from build123d import *

# Parameters (mm, degrees)
SM_BASE_FLANGE_1_DEPTH     = 500
CHAMFER_2_SIZE             = 1
CUT_EXTRUDE_1_DEPTH        = 1012.596757607
PATTERN_CIRCULAR_1_COUNT   = 4
PATTERN_CIRCULAR_1_ANGLE   = 90
F_1_THE_OTHER_WAY_COUNT    = 4
F_1_THE_OTHER_WAY_ANGLE    = 90
CHAMFER_1_SIZE             = 3
HOLE_WIZARD_M61_AT_2_COUNT = 2
HOLE_WIZARD_M61_AT_2_PITCH = 150
HOLE_WIZARD_M61_AT_3_COUNT = 2
HOLE_WIZARD_M61_AT_3_PITCH = 300
HOLE_WIZARD_M61_AT_4_COUNT = 2
HOLE_WIZARD_M61_AT_4_PITCH = 450
HOLE_WIZARD_M61_AT_5_COUNT = 2
HOLE_WIZARD_M61_AT_5_PITCH = 600
HOLE_WIZARD_M61_AT_6_COUNT = 2
HOLE_WIZARD_M61_AT_6_PITCH = 750
HOLE_WIZARD_M61_AT_7_COUNT = 2
HOLE_WIZARD_M61_AT_7_PITCH = 900


# Sheet-metal steps are written as plain solids
with BuildPart() as part:
    # Sketch 2 → Базовая кромка1 (new, symmetric)
    with BuildSketch(Plane.XY):
        with BuildLine():
            Line((100, 95), (100, 0))
            ThreePointArc((100, 0), (0, -100), (-100, 0))
            Line((-100, 0), (-100, 95))
            Line((-100, 95), (-108, 95))
            Line((-108, 95), (-108, 0))
            ThreePointArc((-108, 0), (0, -108), (108, 0))
            Line((108, 0), (108, 95))
            Line((108, 95), (100, 95))
        make_face()
    extrude(amount=SM_BASE_FLANGE_1_DEPTH, both=True)

    # Фаска2
    chamfer_2_edges = [part.edges().sort_by_distance(p)[0] for p in [
        (100, 47.5, 500),
        (0, -100, 500),
        (-100, 47.5, 500),
        (0, -100, -500),
        (100, 47.5, -500),
        (-100, 47.5, -500),
    ]]
    chamfer(chamfer_2_edges, length=CHAMFER_2_SIZE)

    # Эскиз7 → Вырез-Вытянуть1 (cut, symmetric)
    with BuildSketch(Plane.XY.offset(500)):
        Polygon((0, 0), (-4, -102.92230079), (4, -102.92230079), align=None)
    cut_extrude_1 = extrude(amount=CUT_EXTRUDE_1_DEPTH, both=True, mode=Mode.SUBTRACT)

    # Круговой массив1: Вырез-Вытянуть1 ×4 about axis
    pattern_circular_1_axis = Axis((0, 0, 0), (0, 0, -1))
    for i in range(1, PATTERN_CIRCULAR_1_COUNT):
        add(cut_extrude_1.rotate(pattern_circular_1_axis, i * PATTERN_CIRCULAR_1_ANGLE / (PATTERN_CIRCULAR_1_COUNT - 1)), mode=Mode.SUBTRACT)

    # 1 the other way: Вырез-Вытянуть1 ×4 about axis
    f_1_the_other_way_axis = Axis((0, 0, 0), (0, 0, 1))
    for i in range(1, F_1_THE_OTHER_WAY_COUNT):
        add(cut_extrude_1.rotate(f_1_the_other_way_axis, i * F_1_THE_OTHER_WAY_ANGLE / (F_1_THE_OTHER_WAY_COUNT - 1)), mode=Mode.SUBTRACT)

    # Фаска1
    chamfer_1_edges = [part.edges().sort_by_distance(p)[0] for p in [
        (100, 95, 0),
        (-100, 95, 0),
    ]]
    chamfer(chamfer_1_edges, length=CHAMFER_1_SIZE)

    # Эскиз9 → Зенковка для винта с полупотайной головкой M61 (revolve, cut)
    with BuildSketch(Plane(origin=(-100, 75, 450), x_dir=(0, 0, -1), z_dir=(0, 1, 0))):
        Polygon((0, 0), (0, 18.982840043), (3.3, 17), (3.3, 3), (6.3, 0), align=None)
    hole_wizard_m61 = revolve(axis=Axis((-93.65, 75, 450), (-1, 0, 0)), mode=Mode.SUBTRACT)

    # Зенковка для винта с полупотайной головкой M61 at 2: Зенковка для винта с полупотайной головкой M61 ×2
    with Locations(*[(0, 0, -i * HOLE_WIZARD_M61_AT_2_PITCH) for i in range(1, HOLE_WIZARD_M61_AT_2_COUNT)]):
        add(hole_wizard_m61, mode=Mode.SUBTRACT)

    # Зенковка для винта с полупотайной головкой M61 at 3: Зенковка для винта с полупотайной головкой M61 ×2
    with Locations(*[(0, 0, -i * HOLE_WIZARD_M61_AT_3_PITCH) for i in range(1, HOLE_WIZARD_M61_AT_3_COUNT)]):
        add(hole_wizard_m61, mode=Mode.SUBTRACT)

    # Зенковка для винта с полупотайной головкой M61 at 4: Зенковка для винта с полупотайной головкой M61 ×2
    with Locations(*[(0, 0, -i * HOLE_WIZARD_M61_AT_4_PITCH) for i in range(1, HOLE_WIZARD_M61_AT_4_COUNT)]):
        add(hole_wizard_m61, mode=Mode.SUBTRACT)

    # Зенковка для винта с полупотайной головкой M61 at 5: Зенковка для винта с полупотайной головкой M61 ×2
    with Locations(*[(0, 0, -i * HOLE_WIZARD_M61_AT_5_PITCH) for i in range(1, HOLE_WIZARD_M61_AT_5_COUNT)]):
        add(hole_wizard_m61, mode=Mode.SUBTRACT)

    # Зенковка для винта с полупотайной головкой M61 at 6: Зенковка для винта с полупотайной головкой M61 ×2
    with Locations(*[(0, 0, -i * HOLE_WIZARD_M61_AT_6_PITCH) for i in range(1, HOLE_WIZARD_M61_AT_6_COUNT)]):
        add(hole_wizard_m61, mode=Mode.SUBTRACT)

    # Зенковка для винта с полупотайной головкой M61 at 7: Зенковка для винта с полупотайной головкой M61 ×2
    with Locations(*[(0, 0, -i * HOLE_WIZARD_M61_AT_7_PITCH) for i in range(1, HOLE_WIZARD_M61_AT_7_COUNT)]):
        add(hole_wizard_m61, mode=Mode.SUBTRACT)

    # Зеркальное отражение1: Зенковка для винта с полупотайной головкой M61 across plane
    add(hole_wizard_m61.mirror(Plane(origin=(0, 0, 0), x_dir=(0, 0, 1), z_dir=(1, 0, 0))), mode=Mode.SUBTRACT)

    # Зеркальное отражение1 copy 1 sketch → Зеркальное отражение1 copy 1 (revolve, cut)
    with BuildSketch(Plane(origin=(100, 75, 300), x_dir=(0, 0, -1), z_dir=(0, 1, 0))):
        Polygon((0, 0), (0, -18.982840043), (3.3, -17), (3.3, -3), (6.3, 0), align=None)
    revolve(axis=Axis((93.65, 75, 300), (-1, 0, 0)), mode=Mode.SUBTRACT)

    # Зеркальное отражение1 copy 2 sketch → Зеркальное отражение1 copy 2 (revolve, cut)
    with BuildSketch(Plane(origin=(100, 75, 150), x_dir=(0, 0, -1), z_dir=(0, 1, 0))):
        Polygon((0, 0), (0, -18.982840043), (3.3, -17), (3.3, -3), (6.3, 0), align=None)
    revolve(axis=Axis((93.65, 75, 150), (-1, 0, 0)), mode=Mode.SUBTRACT)

    # Зеркальное отражение1 copy 3 sketch → Зеркальное отражение1 copy 3 (revolve, cut)
    with BuildSketch(Plane(origin=(100, 75, 0), x_dir=(0, 0, -1), z_dir=(0, 1, 0))):
        Polygon((0, 0), (0, -18.982840043), (3.3, -17), (3.3, -3), (6.3, 0), align=None)
    revolve(axis=Axis((93.65, 75, 0), (-1, 0, 0)), mode=Mode.SUBTRACT)

    # Зеркальное отражение1 copy 4 sketch → Зеркальное отражение1 copy 4 (revolve, cut)
    with BuildSketch(Plane(origin=(100, 75, -150), x_dir=(0, 0, -1), z_dir=(0, 1, 0))):
        Polygon((0, 0), (0, -18.982840043), (3.3, -17), (3.3, -3), (6.3, 0), align=None)
    revolve(axis=Axis((93.65, 75, -150), (-1, 0, 0)), mode=Mode.SUBTRACT)

    # Зеркальное отражение1 copy 5 sketch → Зеркальное отражение1 copy 5 (revolve, cut)
    with BuildSketch(Plane(origin=(100, 75, -300), x_dir=(0, 0, -1), z_dir=(0, 1, 0))):
        Polygon((0, 0), (0, -18.982840043), (3.3, -17), (3.3, -3), (6.3, 0), align=None)
    revolve(axis=Axis((93.65, 75, -300), (-1, 0, 0)), mode=Mode.SUBTRACT)

    # Зеркальное отражение1 copy 6 sketch → Зеркальное отражение1 copy 6 (revolve, cut)
    with BuildSketch(Plane(origin=(100, 75, -450), x_dir=(0, 0, -1), z_dir=(0, 1, 0))):
        Polygon((0, 0), (0, -18.982840043), (3.3, -17), (3.3, -3), (6.3, 0), align=None)
    revolve(axis=Axis((93.65, 75, -450), (-1, 0, 0)), mode=Mode.SUBTRACT)


solid = part.part
The listing builds one solid part. Answer for the finished solid, in the listing's coordinates (mm). A direction names the side the tool comes from. Round coordinates to 2 decimals unless told otherwise and drop trailing zeros. Order: outer loops, then holes, each group sorted by start corner. A loop starts at its lowest first (then second) coordinate and runs counter-clockwise, first axis right, second up. Notation, with made-up numbers: (-23.5, 49.5) - (19.5, 49.5) arc R25 ccw to (19.5, 73.5) - close; hole circle Ø6 at (28, -19.5). An arc over 180 degrees is marked (long way). Write item = value, one per line. Start each with the question number.
1) Straight lines are drawn through the part: L1, parallel to X at y = 85.5, z = 85.5; L2, parallel to Y at x = -3.5, z = -127.5; L3, parallel to X at y = -88, z = -88.5. For each, find the intervals that lie inside material, in ascending order.
2) For faces 5 (the flat face through (31.5, -96.2, 500)), 6 (the conical face through (71.1, -70.6, 499.2)), 7 (the conical face through (71.1, -70.6, -499.2)), 8 (the flat face through (-100, 47, 7)), determine the directions among +Z, -Z, +X, -X, +Y, -Y from which every point of the face is accessible in a straight line to the end or side of a thin tool.
3) For a pull along X with two mould halves and no side action, classify faces 1 (the flat face through (100, 49, 7)), 2 (the cylindrical face through (-2.375, -107.974, 7)), 3 (the conical face through (-70.6, -71.1, 499.2)), 4 (the flat face through (108, 47, 7)) as released by +X, released by -X, zero draft, split by the parting line, or undercut.
4) Section A-A, the plane y = 16.5 is taken. Write down the section's boundary in (x, z), plus the area to 3 significant figures.
5) Given pin 1 (6.5 mm diameter, centred on x = 0.5, z = 41, fed in from +Y); pin 2 (1 mm diameter, centred on x = 52.5, z = 215.5, fed in from -Y); pin 3 (5 mm diameter, centred on y = -12, z = -28, fed in from +X), each flat-ended and moving along its own axis, determine where each tip first touches the part or whether it passes through.
Results list:
q1.L1 = -108 to -100, 100 to 108
q1.L2 = -107.94 to -102.92
q1.L3 = -62.61 to -53.42, 53.42 to 62.61
q2.face_5 = +Z, +X, -X, +Y, -Y
q2.face_6 = +Z, +Y
q2.face_7 = -Z, +Y
q2.face_8 = +Z, -Z, +Y
q3.face_1 = undercut
q3.face_2 = split by the parting line
q3.face_3 = undercut
q3.face_4 = released by +X
q4.outline = (-108, -500) - (-101, -500) - (-100, -499) - (-100, 499) - (-101, 500) - (-108, 500) - close; (100, -499) - (101, -500) - (108, -500) - (108, 500) - (101, 500) - (100, 499) - close
q4.area = 16,000 mm^2
q5.pin_1 = -102.92
q5.pin_2 = -94.66
q5.pin_3 = 107.58
